Build history of the part. All positions in model axes, mm. A direction names the side the tool comes from. Round coordinates to 2 decimals unless told otherwise and drop trailing zeros. Write each loop counter-clockwise with the first axis right and the second up, starting at its lowest first coordinate (ties: lowest second). Pieces come first, ordered by that corner, then holes. Notation, with made-up numbers: M -10,39.5 L 19,39.5 A35 cw 19,77.5 Z; hole C 61.25,85.5 d8. An arc over 180 degrees is marked long. Write item = value, one per line. Start each with the question number.
Q1. Drop flat-ended pins along their axis: P1, Ø10, axis at y = -812.5, z = 110.5, coming from the +X side; P2, Ø16, axis at y = -362.5, z = 83, coming from the -X side; P3, Ø11.5, axis at x = -25, y = -362.5, coming from the +Z side. Give the stop position or say it passes through.
Q2. Band-saw the part on B-B on z = 55.5. Write the cut outline in (x, y), plus the area to 3 significant figures.
Q3. Probe L1, parallel to X at y = -1062.5, z = 128.65; L2, parallel to Z at x = 3.3, y = -862.5; L3, parallel to Z at x = 3.75, y = -1462.5. List the from-to ranges inside material, lowest first.
Q4. Band-saw the part on A-A on y = -306. Write the cut outline in (x, z).
Q5. Tool access for faces 1 (the flat face through (-29, -752, 0)), 2 (the flat face through (5.8, -1519.2, 73.5)), 3 (the flat face through (45, -752, 124)): list every direction of +Z, -Z, +X, -X, +Y, -Y with a clear straight run to the whole face (end or side of a thin tool).
```python
from build123d import *

# Parameters (mm, degrees)
F1_DEPTH    = 1525
F3_DEPTH    = 136.001
F4_R        = 8
F5_R        = 8
F6_R        = 14
F7_T1_DEPTH = 1583
F8_R        = 4.1
F9_DEPTH    = 136.001
F10_R       = 5
F11_DEPTH   = 76.001
F12_R       = 5
F13_DEPTH   = 6.001
F15_DEPTH   = 136.001
F16_R       = 5


# Not quite as in the source:
# - a fillet or chamfer that OpenCascade refuses, or shapes differently, is made with other operations: its cross-section is extruded or revolved along the edge and cut away or added
# - two fillets or chamfers of one size are made in one step


with BuildPart() as f1:
    # F0 (on Front) → F1 (new body)
    with BuildSketch(Plane.XZ):
        Polygon((0, 130), (0, 0), (-50, 0), (-50, -6), (6, -6), (6, 124), (76, 124), (76, 130), align=None)
    extrude(amount=F1_DEPTH)

    # F2 (on face) → F3 (cut, through all)
    with BuildSketch(Plane.XY.offset(130)):
        Polygon((76, -76), (76, 0), (0, 0), align=None)
        Polygon((76, -1525), (76, -1449), (0, -1525), align=None)
    extrude(amount=-F3_DEPTH, mode=Mode.SUBTRACT)

    # F4
    f4_edges = [f1.edges().sort_by_distance(p)[0] for p in [
        (6, -762.5, 124),
    ]]
    fillet(f4_edges, radius=F4_R)

    # F5
    f5_edges = [f1.edges().sort_by_distance(p)[0] for p in [
        (0, -762.5, 0),
    ]]
    fillet(f5_edges, radius=F5_R)

    # F6
    f6_edges = [f1.edges().sort_by_distance(p)[0] for p in [
        (0, -762.5, 130),
    ]]
    fillet(f6_edges, radius=F6_R)

    # F7: fillet of radius 14 on 1 edges, made by hand

    # F7_s2 → F7_t1 (cut)
    with BuildSketch(Plane.XZ.offset(-29)):
        with BuildLine():
            ThreePointArc((-8, -6), (1.8994949366, -1.8994949366), (6, 8))
            Line((6, 8), (6, -6))
            Line((6, -6), (-8, -6))
        make_face()
    extrude(amount=F7_T1_DEPTH, mode=Mode.SUBTRACT)

    # F8 (on face) → F9 (cut, through all)
    with BuildSketch(Plane.XY.offset(130)):
        with Locations((51, -1362.5)):
            Circle(F8_R)
        with Locations((51, -1262.5)):
            Circle(F8_R)
        with Locations((51, -1162.5)):
            Circle(F8_R)
        with Locations((51, -1062.5)):
            Circle(F8_R)
        with Locations((51, -962.5)):
            Circle(F8_R)
        with Locations((51, -862.5)):
            Circle(F8_R)
        with Locations((51, -762.5)):
            Circle(F8_R)
        with Locations((51, -662.5)):
            Circle(F8_R)
        with Locations((51, -562.5)):
            Circle(F8_R)
        with Locations((51, -462.5)):
            Circle(F8_R)
        with Locations((51, -362.5)):
            Circle(F8_R)
        with Locations((51, -262.5)):
            Circle(F8_R)
        with Locations((51, -162.5)):
            Circle(F8_R)
    extrude(amount=-F9_DEPTH, mode=Mode.SUBTRACT)

    # F10 (on face) → F11 (cut, through all)
    with BuildSketch(Plane(origin=(0, 0, 0), x_dir=(0, -1, 0), z_dir=(-1, 0, 0))):
        with Locations((1462.5, 33)):
            Circle(F10_R)
        with Locations((1362.5, 33)):
            Circle(F10_R)
        with Locations((1262.5, 33)):
            Circle(F10_R)
        with Locations((1162.5, 33)):
            Circle(F10_R)
        with Locations((1062.5, 33)):
            Circle(F10_R)
        with Locations((962.5, 33)):
            Circle(F10_R)
        with Locations((862.5, 33)):
            Circle(F10_R)
        with Locations((762.5, 33)):
            Circle(F10_R)
        with Locations((662.5, 33)):
            Circle(F10_R)
        with Locations((562.5, 33)):
            Circle(F10_R)
        with Locations((462.5, 33)):
            Circle(F10_R)
        with Locations((362.5, 33)):
            Circle(F10_R)
        with Locations((262.5, 33)):
            Circle(F10_R)
        with Locations((162.5, 33)):
            Circle(F10_R)
        with Locations((62.5, 33)):
            Circle(F10_R)
        with Locations((1462.5, 83)):
            Circle(F10_R)
        with Locations((1362.5, 83)):
            Circle(F10_R)
        with Locations((1262.5, 83)):
            Circle(F10_R)
        with Locations((1162.5, 83)):
            Circle(F10_R)
        with Locations((1062.5, 83)):
            Circle(F10_R)
        with Locations((962.5, 83)):
            Circle(F10_R)
        with Locations((862.5, 83)):
            Circle(F10_R)
        with Locations((462.5, 83)):
            Circle(F10_R)
        with Locations((562.5, 83)):
            Circle(F10_R)
        with Locations((662.5, 83)):
            Circle(F10_R)
        with Locations((762.5, 83)):
            Circle(F10_R)
        with Locations((162.5, 83)):
            Circle(F10_R)
        with Locations((262.5, 83)):
            Circle(F10_R)
        with Locations((62.5, 83)):
            Circle(F10_R)
        with Locations((362.5, 83)):
            Circle(F10_R)
    extrude(amount=-F11_DEPTH, mode=Mode.SUBTRACT)

    # F12 (on face) → F13 (cut, through all)
    with BuildSketch(Plane.XY):
        with Locations((-25, -1462.5)):
            Circle(F12_R)
        with Locations((-25, -1362.5)):
            Circle(F12_R)
        with Locations((-25, -1262.5)):
            Circle(F12_R)
        with Locations((-25, -1162.5)):
            Circle(F12_R)
        with Locations((-25, -1062.5)):
            Circle(F12_R)
        with Locations((-25, -962.5)):
            Circle(F12_R)
        with Locations((-25, -862.5)):
            Circle(F12_R)
        with Locations((-25, -762.5)):
            Circle(F12_R)
        with Locations((-25, -662.5)):
            Circle(F12_R)
        with Locations((-25, -562.5)):
            Circle(F12_R)
        with Locations((-25, -462.5)):
            Circle(F12_R)
        with Locations((-25, -362.5)):
            Circle(F12_R)
        with Locations((-25, -262.5)):
            Circle(F12_R)
        with Locations((-25, -162.5)):
            Circle(F12_R)
        with Locations((-25, -62.5)):
            Circle(F12_R)
    extrude(amount=-F13_DEPTH, mode=Mode.SUBTRACT)

    # F14 (on face) → F15 (cut, through all)
    with BuildSketch(Plane.XY.offset(130)):
        Polygon((76, -76), (36, -36), (36, -62.5), (51.186291501, -62.5), (76, -87.313708499), align=None)
        Polygon((36, -1462.5), (36, -1489), (76, -1449), (76, -1437.686291501), (51.186291501, -1462.5), align=None)
    extrude(amount=-F15_DEPTH, mode=Mode.SUBTRACT)

    # F16
    f16_edges = [f1.edges().sort_by_distance(p)[0] for p in [
        (36, -36, 127),
        (36, -62.5, 127),
        (36, -1489, 127),
        (36, -1462.5, 127),
        (51.186292, -62.5, 127),
        (76, -87.313708, 127),
        (51.186292, -1462.5, 127),
        (76, -1437.686292, 127),
        (-50, 0, -3),
        (-50, -1525, -3),
    ]]
    fillet(f16_edges, radius=F16_R)


solid = f1.part
```
Conclusion:
q1.P1 = 6
q1.P2 = 0
q1.P3 = 0
q2.outline = M 0,-1525 L 6,-1519 L 6,-6 L 0,0 Z
q2.area = 9,110 mm^2
q3.L1 = 8 to 46.9, 55.1 to 76
q3.L2 = -0.26 to 28, 38 to 78, 88 to 125.03
q3.L3 = 0.39 to 28, 38 to 78, 88 to 125.54
q4.outline = M -50,-6 L -8,-6 A14 ccw 6,8 L 6,116 A8 cw 14,124 L 76,124 L 76,130 L 14,130 A14 ccw 0,116 L 0,8 A8 cw -8,0 L -50,0 Z
q5.face_1 = +Z, -X, +Y, -Y
q5.face_2 = +Z, -Z, +X, -Y
q5.face_3 = -Z, +X, +Y, -Y
